Answer from the drawing. Dimensions are ordinates in mm from the lowest x, y and z of the part. A direction names the side the tool comes from. Give positions to 0.01 mm unless a question says otherwise; leave off trailing zeros. Write each loop counter-clockwise with the first axis right and the second up, starting at its lowest first coordinate (ties: lowest second). Pieces come first, ordered by that corner, then holes. Notation, with made-up numbers: M 29,54.5 L 62,54.5 A21 ccw 62,59.5 Z; hole C 88,65 d11. An arc over 180 degrees is marked long. Answer as a JSON object with one key per item and string values.
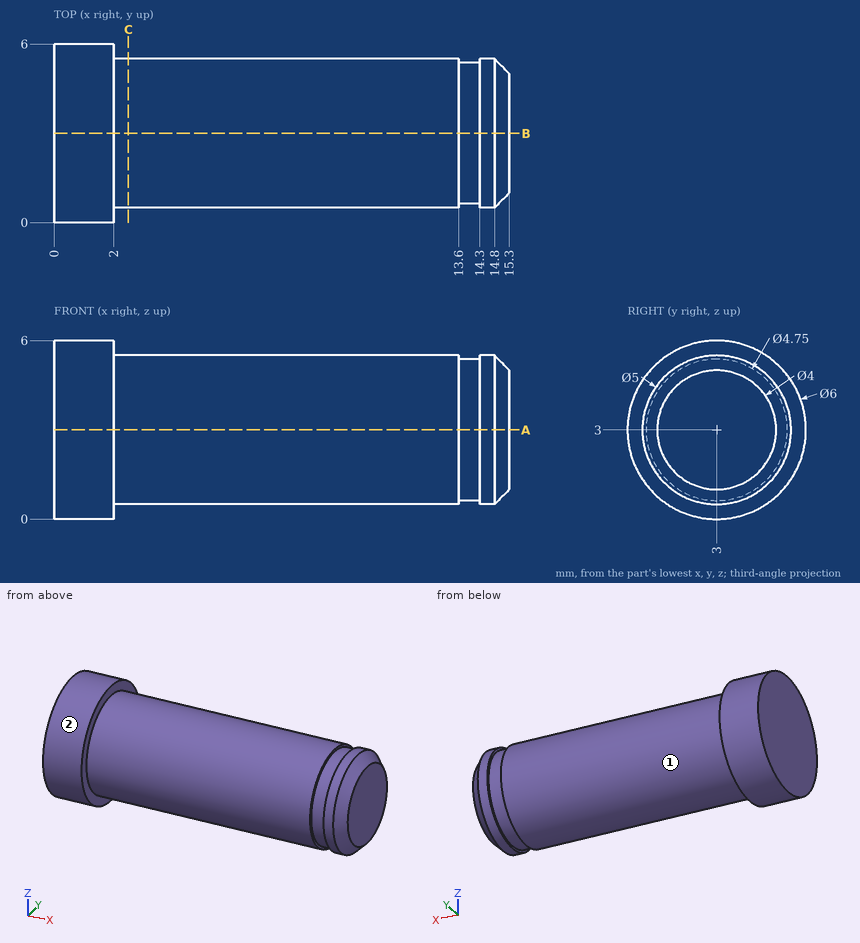
1. A cutting plane is placed at A-A, the plane z = 3. Give the vertices of the cut face in (x, y) (3 decimals).
Verdict:
{"outline": "M 0,0 L 2,0 L 2,0.5 L 13.6,0.5 L 13.6,0.625 L 14.3,0.625 L 14.3,0.5 L 14.8,0.5 L 15.3,1 L 15.3,5 L 14.8,5.5 L 14.3,5.5 L 14.3,5.375 L 13.6,5.375 L 13.6,5.5 L 2,5.5 L 2,6 L 0,6 Z"}
2. For the marked faces 1 and 2, determine the directions among +Z, -Z, +X, -X, +Y, -Y from which every point of the face is accessible in a straight line to the end or side of a thin tool.
Verdict:
{"face 1": "+X", "face 2": "+X, -X"}
3. A cutting plane is placed at C-C, the plane x = 2.5. Give the vertices of the cut face in (y, z).
Verdict:
{"outline": "C 3,3 d5"}
4. Consider line 1 along X through (y, z) = (0.35, 3.7); line 2 along X through (y, z) = (5.4, 3.5); line 3 along Y through (x, z) = (5.75, 3.95). Determine where each line is inside the solid, lowest interval first.
Verdict:
{"line 1": "x = 0 to 2", "line 2": "x = 0 to 13.6, 14.3 to 14.85", "line 3": "y = 0.69 to 5.31"}
5. Flat-ended cylindrical pins translate along their axes: pin 1 (1.5 mm diameter, centred on x = 9.5, y = 5.5, fed in from -Z); pin 2 (1.5 mm diameter, centred on x = 12, z = 2.5, fed in from +Y). Find the tip coordinate at first contact, or state that the pin passes through.
Verdict:
{"pin 1": "stops at z = 1.21", "pin 2": "stops at y = 5.5"}
